CAD build for the part. Positions are in the model's coordinates, mm. Coordinates: 2 decimals unless noted, no trailing zeros. Write each loop counter-clockwise with the first axis right and the second up, starting at its lowest first coordinate (ties: lowest second). Pieces come first, ordered by that corner, then holes. Notation, with made-up numbers: (78.5, 41.25) - (89.5, 41.25) arc R20 ccw to (89.5, 55.25) - close; hole circle Ø8 at (29.25, -14). An arc over 180 degrees is marked (long way). Answer in a Markdown table with one row per item. Add a question column.
Q1. Two-plate mould, pull along X, no slides. Class faces 1 (the flat face through (-12.5, -1, 3)), 2 (the cylindrical face through (-0.573, 32.437, 3.451)), 3 (the flat face through (12.5, -1, 3)): +X half, -X half, draft (parallel to the pull), parting line (faces both ways), or undercut.
Q2. Band-saw the part on B-B (z = 104.5). List the corners of the cut face in (x, y), and give its area (3 significant figures).
Q3. Drill centre lines: line 1 along X through (y, z) = (-35, 1.75); line 2 along Z through (x, y) = (3, 15); line 3 along X through (y, z) = (-34, 88). Where is each one in solid material? Low to high. Write a range as from..to.
Q4. Pin check, flat tips, straight feed: pin 1 (3.5 mm diameter, centred on y = 18.5, z = 2.5, fed in from +X); pin 2 (4.5 mm diameter, centred on x = 0, y = 35, fed in from +Z); pin 3 (6 mm diameter, centred on y = -18.5, z = 124, fed in from +X); pin 4 (3 mm diameter, centred on y = 20, z = 100, fed in from -X). Stop position of each tip, or through.
Q5. Band-saw the part on C-C (x = -8). List the corners of the cut face in (y, z), and give its area (3 significant figures).
```python
from build123d import *

# Parameters (mm, degrees)
SKETCH_W        = 25
SKETCH_H        = 80
PAD_DEPTH       = 7
SKETCH001_R     = 2.625
POCKET_DEPTH    = 8
SKETCH002_W     = 8
SKETCH002_H     = 80
PAD001_DEPTH    = 145
SKETCH003_W     = 25
SKETCH003_H     = 80
PAD002_DEPTH    = 6
SKETCH004_R     = 2.2
POCKET001_DEPTH = 7


with BuildPart() as part:
    # Sketch → Pad (new body)
    with BuildSketch(Plane.XY):
        Rectangle(SKETCH_W, SKETCH_H)
    extrude(amount=PAD_DEPTH)

    # Sketch001 → Pocket (cut)
    with BuildSketch(Plane.XY):
        with Locations((-0.003934, 35)):
            Circle(SKETCH001_R)
        with Locations((-0.004048, -35)):
            Circle(SKETCH001_R)
    extrude(amount=POCKET_DEPTH, mode=Mode.SUBTRACT)

    # Sketch002 → Pad001 (join)
    with BuildSketch(Plane.XY):
        with Locations((8.398357, 0)):
            Rectangle(SKETCH002_W, SKETCH002_H)
    extrude(amount=PAD001_DEPTH)

    # Sketch003 (on Face18 of Pad001) → Pad002 (join)
    with BuildSketch(Plane.XY.offset(145)):
        with Locations((16.875703, 0)):
            Rectangle(SKETCH003_W, SKETCH003_H)
    extrude(amount=PAD002_DEPTH)

    # Sketch004 (on Face7 of Pad002) → Pocket001 (cut)
    with BuildSketch(Plane.XY.offset(151)):
        with Locations((23, 33)):
            Circle(SKETCH004_R)
        with Locations((23, -33)):
            Circle(SKETCH004_R)
    extrude(amount=-POCKET001_DEPTH, mode=Mode.SUBTRACT)


solid = part.part
```
Checked values:
| question | item | result |
|---|---|---|
| 1 | face 1 | -X half |
| 1 | face 2 | undercut |
| 1 | face 3 | +X half |
| 2 | outline | (4.4, -40) - (12.4, -40) - (12.4, 40) - (4.4, 40) - close |
| 2 | area | 640 mm² |
| 3 | line 1 | x = -12.5..-2.63, 2.62..12.5 |
| 3 | line 2 | z = 0..7 |
| 3 | line 3 | x = 4.4..12.4 |
| 4 | pin 1 | stops at x = 12.5 |
| 4 | pin 2 | passes through |
| 4 | pin 3 | stops at x = 12.4 |
| 4 | pin 4 | stops at x = 4.4 |
| 5 | outline | (-40, 0) - (40, 0) - (40, 7) - (-40, 7) - close |
| 5 | area | 560 mm² |
